Source: CAD feature listing. Evaluate the final solid. Frame: model axes, mm. Give positions to 0.01 mm unless a question says otherwise; leave off trailing zeros. Order: outer loops, then holes, each group sorted by start corner. A loop starts at its lowest first (then second) coordinate and runs counter-clockwise, first axis right, second up. Notation, with made-up numbers: M 26,66 L 41,66 A17 cw 41,77 Z; hole C 58,-4.75 d5. An arc over 180 degrees is marked long. Answer in a Markdown table with one row per item. Add a question column.
(1) Section query C-C, the plane y = 80. Return loops of the section in (x, z), plus the area to 3 significant figures.
(2) Section query B-B, the plane x = 16.5. Return loops of the section in (y, z), plus the area to 3 significant figures.
(3) Section query A-A, the plane z = 6. Return loops of the section in (x, y).
(4) Material intervals for line 1 along Y through (x, z) = (55, 3.75); line 2 along X through (y, z) = (50.5, 5.25); line 3 along X through (y, z) = (38, 4.75), sorted ascending.
from build123d import *

# Parameters (mm, degrees)
Y_KSEKLIK_EKSTR_ZYON1_DEPTH = 8


with BuildPart() as part:
    # Çizim1 → Yükseklik-Ekstrüzyon1 (new body)
    with BuildSketch(Plane.XY):
        with BuildLine():
            Line((0, 15), (0, 0))
            Line((0, 0), (131, 0))
            Line((131, 0), (131, 109))
            Line((131, 109), (79, 109))
            Line((79, 109), (13.510611656, 45.388360721))
            ThreePointArc((13.510611656, 45.388360721), (5.385413078, 30.803232265), (0, 15))
        make_face()
    extrude(amount=Y_KSEKLIK_EKSTR_ZYON1_DEPTH)


solid = part.part
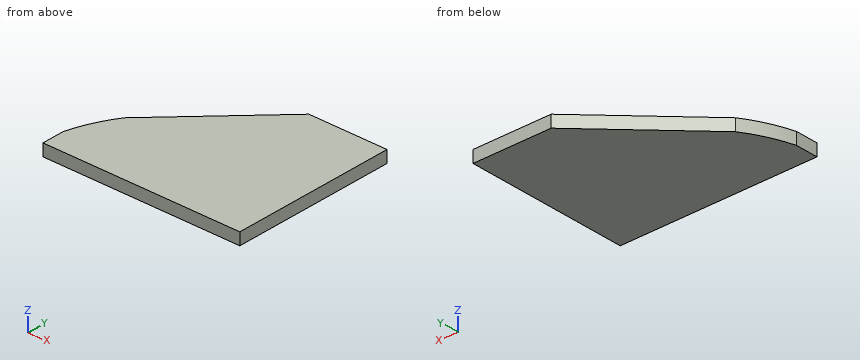
Values follow:
| question | item | result |
|---|---|---|
| 1 | outline | M 49.14,0 L 131,0 L 131,8 L 49.14,8 Z |
| 1 | area | 655 mm² |
| 2 | outline | M 0,0 L 48.29,0 L 48.29,8 L 0,8 Z |
| 2 | area | 386 mm² |
| 3 | outline | M 0,0 L 131,0 L 131,109 L 79,109 L 13.51,45.39 A92.97 ccw 0,15 Z |
| 4 | line 1 | y = 0 to 85.69 |
| 4 | line 2 | x = 18.77 to 131 |
| 4 | line 3 | x = 8.97 to 131 |
